Can you work these out from the model? Positions are in its coordinate system, mm. Round coordinates to 2 decimals unless told otherwise and drop trailing zeros. Order: outer loops, then holes, each group sorted by start corner. A loop starts at its lowest first (then second) coordinate and runs counter-clockwise, first axis right, second up. Notation, with made-up numbers: M -37,55 L -31,55 A12 cw -31,62 Z; hole C 11.25,63 d2. An arc over 180 degrees is marked long. Answer as a JSON object with one key per item and string values. Group by question number.
Autodesk Inventor part; units mm, degrees
ref_plane "YZ Plane" through (0, 0, 0) normal (1, 0, 0) x (0, 1, 0)
ref_plane "XZ Plane" through (0, 0, 0) normal (0, 1, 0) x (-1, 0, 0)
ref_plane "XY Plane" through (0, 0, 0) normal (0, 0, 1) x (1, 0, 0)
sketch "Эскиз1" plane through (0, 0, 0) normal (0, 0, 1) x (1, 0, 0)
  line L0 (-30, 21.6) -> (30, 21.6)
  line L1 (30, 21.6) -> (30, -21.6)
  line L2 (30, -21.6) -> (-30, -21.6)
  line L3 (-30, -21.6) -> (-30, 21.6)
  line L4 (-30, 21.6) -> (30, -21.6) construction
  line L5 (30, 21.6) -> (-30, -21.6) construction
  point P0 (0, 0)
  dimension "d0" = 60
  dimension "d1" = 43.2
extrude "Выдавливание1" add sketch "Эскиз1" along normal blind 4
sketch "Эскиз2" plane through (0, 0, 0) normal (0, 0, -1) x (-1, 0, 0)
  line L0 (-12.5, -9) -> (12.5, -9) construction
  line L1 (0, 0) -> (0, -21.6) construction
  line L2 (30, -21.6) -> (-30, -21.6)
  circle A0 centre (-12.5, -9) radius 1.6
  circle A1 centre (12.5, -9) radius 1.6
  line L3 (-30, -21.6) -> (-30, 21.6)
  line L4 (-30, 0) -> (30, 0) construction
  line L5 (30, 21.6) -> (30, -21.6)
  point P0 (0, -9)
  dimension "d4" = 25
  dimension "d5" = 3.2
  dimension "d6" = 3.2
  dimension "d7" = 9
extrude "Выдавливание2" cut sketch "Эскиз2" against normal blind 4
sketch "Эскиз3" plane through (0, 0, 0) normal (0, 0, -1) x (-1, 0, 0)
  circle A0 centre (-25.5, 8.4) radius 1.75 construction
  circle A1 centre (25.5, 8.4) radius 1.75 construction
  circle A2 centre (25.5, -11.6) radius 1.75 construction
  circle A3 centre (-25.5, -11.6) radius 1.75 construction
  circle A4 centre (-25.5, 8.4) radius 1.6
  circle A5 centre (25.5, 8.4) radius 1.6
  circle A6 centre (-25.5, -11.6) radius 1.6
  circle A7 centre (25.5, -11.6) radius 1.6
  point P0 (0, 0)
  dimension "d10" = 3.2
  dimension "d11" = 3.2
  dimension "d12" = 3.2
  dimension "d13" = 3.2
extrude "Выдавливание3" cut sketch "Эскиз3" against normal blind 10
sketch "Эскиз4" plane through (0, 0, 0) normal (0, 0, -1) x (-1, 0, 0)
  line L0 (-30, 21.6) -> (30, 21.6) construction
  line L1 (-30, 21.6) -> (30, 21.6)
  line L2 (-30, 21.6) -> (30, 21.6)
  line L3 (30, 21.6) -> (30, 39.6)
  line L4 (30, 39.6) -> (-30, 39.6)
  line L5 (-30, 39.6) -> (-30, 21.6)
  dimension "d18" = 60
  dimension "d19" = 18
extrude "Выдавливание4" add sketch "Эскиз4" against normal blind 4
sketch "Эскиз5" plane through (0, 0, 0) normal (0, 0, -1) x (-1, 0, 0)
  line L0 (-11.55, 23.6) -> (11.45, 23.6) construction
  line L1 (11.45, 23.6) -> (11.45, 35.6) construction
  line L2 (-11.55, 23.6) -> (11.45, 35.6) construction
  line L3 (-16.55, 36.6) -> (16.45, 36.6)
  line L4 (16.45, 36.6) -> (16.45, 22.6)
  line L5 (16.45, 22.6) -> (-16.55, 22.6)
  line L6 (-16.55, 22.6) -> (-16.55, 36.6)
  line L7 (-16.55, 36.6) -> (16.45, 22.6) construction
  line L8 (16.45, 36.6) -> (-16.55, 22.6) construction
  point P0 (0, 0)
  point P1 (-0.05, 29.6)
  dimension "d22" = 1
  dimension "d23" = 5
extrude "Выдавливание5" cut sketch "Эскиз5" against normal blind 4
sketch "Эскиз6" plane through (0, 0, 4) normal (0, 0, 1) x (1, 0, 0)
  line L0 (11.7, 17.6) -> (11.7, 21.6) construction
  line L1 (11.7, 21.6) -> (30, 21.6) construction
  line L2 (30, 21.6) -> (30, 17.6) construction
  line L3 (30, 17.6) -> (11.7, 17.6) construction
  line L4 (-8.3, 17.6) -> (-8.3, 21.6) construction
  line L5 (-8.3, 21.6) -> (8.3, 21.6) construction
  line L6 (8.3, 21.6) -> (8.3, 17.6) construction
  line L7 (8.3, 17.6) -> (-8.3, 17.6) construction
  line L8 (-11.7, 21.6) -> (-11.7, 17.6) construction
  line L9 (-11.7, 17.6) -> (-30, 17.6) construction
  line L10 (-30, 17.6) -> (-30, 21.6) construction
  line L11 (-30, 21.6) -> (-11.7, 21.6) construction
  line L12 (11.7, 21.6) -> (8.3, 17.6) construction
  line L13 (-8.3, 21.6) -> (-11.7, 17.6) construction
  circle A0 centre (-10, 19.6) radius 1.6
  circle A1 centre (10, 19.6) radius 1.6
  point P0 (0, 0)
  dimension "d26" = 3.2
  dimension "d27" = 3.2
extrude "Выдавливание6" cut sketch "Эскиз6" against normal blind 10
sketch "Эскиз7" plane through (0, 0, 0) normal (0, 0, -1) x (-1, 0, 0)
  line L0 (-10, -21.6) -> (-13.3, -21.6)
  line L1 (-13.3, -21.6) -> (-13.3, -13.6)
  line L2 (-13.3, -13.6) -> (-10, -13.6)
  line L3 (-10, -13.6) -> (-10, -21.6)
  line L4 (-20, -21.6) -> (20, -21.6)
  line L5 (30, -21.6) -> (-30, -21.6)
  line L6 (-8.9, -17.6) -> (-14.4, -17.6)
  line L7 (-14.4, -17.6) -> (-14.4, -15.3)
  line L8 (-14.4, -15.3) -> (-8.9, -15.3)
  line L9 (-8.9, -15.3) -> (-8.9, -17.6)
  line L10 (-11.65, -13.6) -> (-11.65, -21.6) construction
  line L11 (0, -21.6) -> (0, -16.45)
  line L12 (10, -21.6) -> (13.3, -21.6)
  line L13 (13.3, -21.6) -> (13.3, -13.6)
  line L14 (13.3, -13.6) -> (10, -13.6)
  line L15 (10, -13.6) -> (10, -21.6)
  line L16 (8.9, -17.6) -> (14.4, -17.6)
  line L17 (14.4, -17.6) -> (14.4, -15.3)
  line L18 (14.4, -15.3) -> (8.9, -15.3)
  line L19 (8.9, -15.3) -> (8.9, -17.6)
  line L20 (11.65, -13.6) -> (11.65, -21.6) construction
  point P0 (0, 0)
  point P1 (-11.65, -15.3)
  point P2 (11.65, -15.3)
  point P3 (-13.3, -17.6)
  point P4 (-10, -17.6)
  point P5 (-10, -15.3)
  point P6 (-13.3, -15.3)
  point P7 (13.3, -15.3)
  point P8 (10, -15.3)
  point P9 (10, -17.6)
  point P10 (10, -21.6)
  point P11 (13.3, -21.6)
  point P12 (13.3, -17.6)
  dimension "d30" = 3.3
  dimension "d31" = 8
  dimension "d32" = 10
  dimension "d33" = 5.5
  dimension "d34" = 2.3
  dimension "d35" = 4
extrude "Выдавливание7" cut sketch "Эскиз7" against normal blind 4
properties part number "стена_для_рельс"
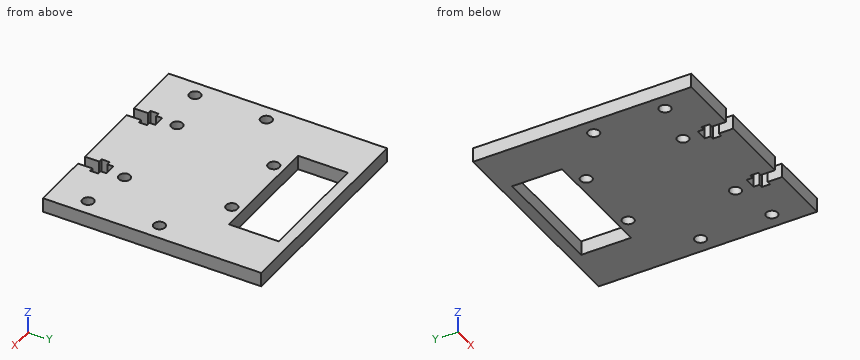
Item 1: I need wall thicknesses on line 1 (Y direction, x = -25.5, z = 2.7); line 2 (Y direction, x = 1, z = 0.5); line 3 (Y direction, x = 12.5, z = 1.6). Which ranges of each line are inside material? Lowest first, please.
Item 2: Suppose I cut it at A-A, the plane x = 6.5. Write out the boundary of the cut face in (y, z), and give its area (3 significant figures).
Item 3: I'm going to push a flat-ended pin straight in: pin 1 Ø5 at (x, y) = (12.5, -9) entering from +Z. Where does the tip first touch, or does it pass through?
Item 4: Suppose I cut it at B-B, the plane y = -16. Write out the boundary of the cut face in (x, z), and give its area (3 significant figures).
Item 5: Suppose I cut it at C-C, the plane x = -25.5. Write out the boundary of the cut face in (y, z), and give its area (3 significant figures).
Item 6: Suppose I cut it at D-D, the plane y = 33. Write out the boundary of the cut face in (x, z).
Computed:
{
 "1": {"line 1": "y = -21.6 to -13.2, -10 to 6.8, 10 to 39.6", "line 2": "y = -21.6 to 22.6, 36.6 to 39.6", "line 3": "y = -13.6 to -10.6, -7.4 to 22.6, 36.6 to 39.6"},
 "2": {"outline": "M -21.6,0 L 22.6,0 L 22.6,4 L -21.6,4 Z; M 36.6,0 L 39.6,0 L 39.6,4 L 36.6,4 Z", "area": "189 mm^2"},
 "3": {"pin 1": "stops at z = 4"},
 "4": {"outline": "M -30,0 L -14.4,0 L -14.4,4 L -30,4 Z; M -8.9,0 L 8.9,0 L 8.9,4 L -8.9,4 Z; M 14.4,0 L 30,0 L 30,4 L 14.4,4 Z", "area": "196 mm^2"},
 "5": {"outline": "M -21.6,0 L -13.2,0 L -13.2,4 L -21.6,4 Z; M -10,0 L 6.8,0 L 6.8,4 L -10,4 Z; M 10,0 L 39.6,0 L 39.6,4 L 10,4 Z", "area": "219 mm^2"},
 "6": {"outline": "M -30,0 L -16.45,0 L -16.45,4 L -30,4 Z; M 16.55,0 L 30,0 L 30,4 L 16.55,4 Z"}
}
